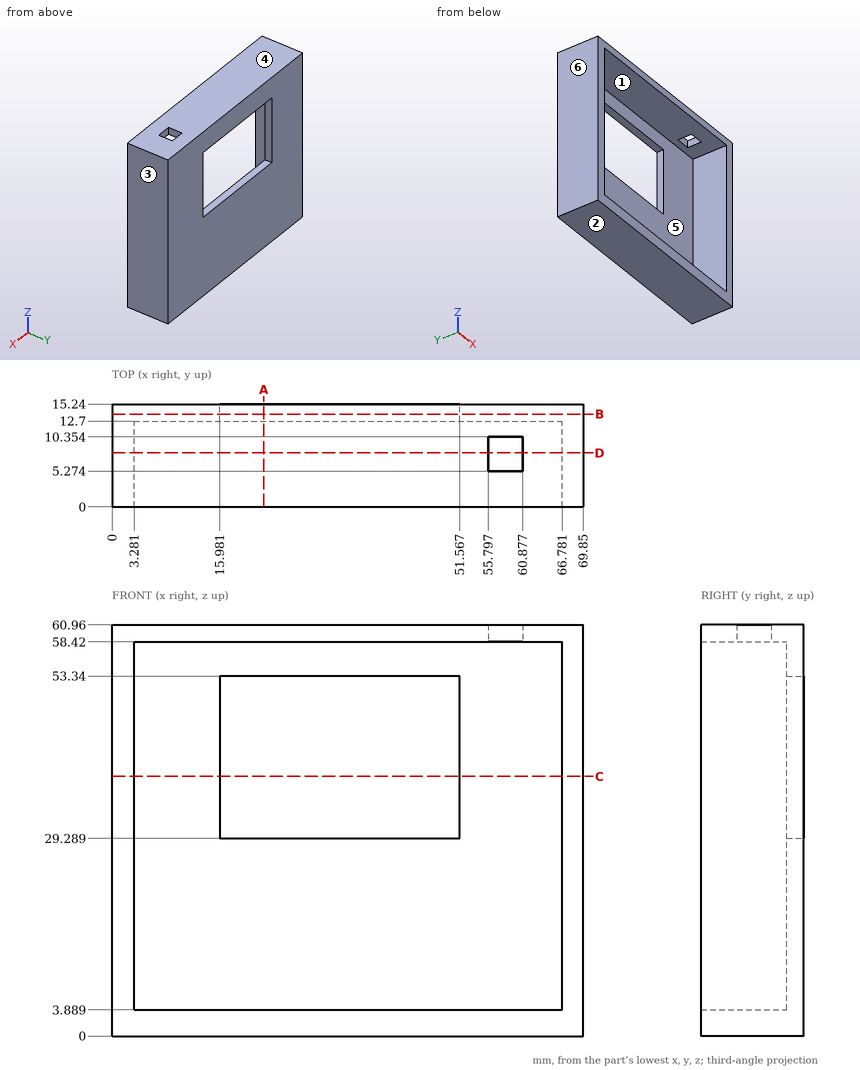
For this review, use the dimensioned drawing (mm, ordinates from the lowest corner) and the shaded views. A direction names the side the tool comes from. Give positions to 0.01 mm unless a question says otherwise; leave off trailing zeros. Loops run counter-clockwise (first coordinate to the right, second up) from the corner with the lowest first, then second, coordinate; pieces in that order, holes last. Notation, with made-up numbers: (18.5, 24.5) - (43.5, 24.5) arc R20 ccw to (43.5, 30.5) - close; hole circle Ø6 at (49, 9). An arc over 180 degrees is marked (long way). Write each question's results on one line, items separated by ' | '.
(1) Take a section at B-B (y = 13.75). Give the boundary of the cut face in (x, z).
Conclusion:
outline: (0, 0) - (69.85, 0) - (69.85, 60.96) - (0, 60.96) - close; hole (15.98, 29.29) - (51.57, 29.29) - (51.57, 53.34) - (15.98, 53.34) - close
(2) For the marked faces 1 and 2, list the 3-axis set-ups (+Z, -Z, +X, -X, +Y, -Y) from which the entire face can be reached by the end or side of a thin tool; tool diameter is ignored.
Conclusion:
face 1: -Y | face 2: -Z, +X, -X, +Y, -Y
(3) Draft analysis for pull direction X (two halves, no side actions). For the marked faces 3, 4, 5 and 6, state which applies: +X half, -X half, draft (parallel to the pull), parting line (faces both ways), or undercut.
Conclusion:
face 3: +X half | face 4: draft | face 5: undercut | face 6: -X half
(4) Take a section at C-C (z = 38.5). Give the boundary of the cut face in (x, y), then the cut area to 3 significant figures.
Conclusion:
outline: (0, 0) - (3.28, 0) - (3.28, 12.7) - (15.98, 12.7) - (15.98, 15.24) - (0, 15.24) - close; (51.57, 12.7) - (66.78, 12.7) - (66.78, 0) - (69.85, 0) - (69.85, 15.24) - (51.57, 15.24) - close | area: 168 mm^2
(5) For line 1 along Z through (x, y) = (16, 1.5); line 2 along X through (y, z) = (11.5, 44); line 3 along Z through (x, y) = (46.5, 13.5), list the stretches that pass through material, from the lowest coordinate up.
Conclusion:
line 1: 0 to 3.89, 58.42 to 60.96 | line 2: 0 to 3.28, 66.78 to 69.85 | line 3: 0 to 29.29, 53.34 to 60.96
(6) Take a section at D-D (y = 8). Give the boundary of the cut face in (x, z).
Conclusion:
outline: (0, 0) - (69.85, 0) - (69.85, 60.96) - (60.88, 60.96) - (60.88, 58.42) - (66.78, 58.42) - (66.78, 3.89) - (3.28, 3.89) - (3.28, 58.42) - (55.8, 58.42) - (55.8, 60.96) - (0, 60.96) - close
(7) For pin 1 Ø3 at (x, z) = (58, 59.5) entering from -Y, flat-tipped, find the tip position at first contact; note if it passes through.
Conclusion:
pin 1: y = 0
(8) Take a section at A-A (x = 22.5). Give the boundary of the cut face in (y, z).
Conclusion:
outline: (0, 0) - (15.24, 0) - (15.24, 29.29) - (12.7, 29.29) - (12.7, 3.89) - (0, 3.89) - close; (0, 58.42) - (12.7, 58.42) - (12.7, 53.34) - (15.24, 53.34) - (15.24, 60.96) - (0, 60.96) - close
